The model under review builds one solid part; all positions refer to its coordinate system, in mm. A direction names the side the tool comes from. Round coordinates to 2 decimals unless told otherwise and drop trailing zeros. Loops run counter-clockwise (first coordinate to the right, second up) from the corner with the lowest first, then second, coordinate; pieces in that order, holes last. Notation, with made-up numbers: (22, -29.5) -> (30, -29.5) arc R30 cw to (30, 4.5) -> close; hole circle Ø8 at (81.25, -39). An arc over 180 degrees is marked (long way). Write each question's results on one line, items separated by ' | '. Start each with the question number.
Item 1: Tool access review of faces 4 (the flat face through (0, -10.9, 5)), 5 (the flat face through (0, -15.9, 3)), 6 (the flat face through (11, -12, 0)), 7 (the cylindrical face through (33.831, -23.126, -13.546)): name each direction out of +Z, -Z, +X, -X, +Y, -Y from which nothing blocks a thin tool from reaching the whole face with its end or side.
Item 2: Clearance check with flat-ended pins moving along their axes: pin 1 Ø2 at (x, y) = (26, 6) entering from +Z; pin 2 Ø3.5 at (x, y) = (-24.89, -5) entering from -Z; pin 3 Ø6 at (x, y) = (2.5, -14) entering from +Z; pin 4 Ø8 at (x, y) = (6, 4.5) entering from -Z. State where each tip first meets the part, or that it passes through.
Item 3: We need section D-D (x = 44). Give the boundary of the cut face in (y, z), and give its area (3 significant figures).
Item 4: Mouldability with a two-part tool opening along Z and no side actions: class faces 1 (the flat face through (-24, -7, 4)), 2 (the cylindrical face through (33.831, -23.126, 31.754)), 3 (the flat face through (2, -14.2, -3)) as pulls with the +Z half, pulls with the -Z half, needs draft (parallel to the pull), parting line crosses it, or undercut.
Item 5: We need section C-C (y = 12.5). Give the boundary of the cut face in (x, z), and give its area (3 significant figures).
Item 6: We need section B-B (x = 24.89). Give the boundary of the cut face in (y, z), and give its area (3 significant figures).
Item 7: We need section A-A (x = -9.5). Give the boundary of the cut face in (y, z).
Item 8: For L1, parallel to Y at x = 24.89, z = 5.7; L2, parallel to Y at x = -24.89, z = 3.25; L3, parallel to Z at x = 45, y = 3, list the stretches that pass through material, from the lowest coordinate up. Write a range as from..to.
Autodesk Inventor part; units mm, degrees
ref_plane "YZ Plane" through (0, 0, 0) normal (1, 0, 0) x (0, 1, 0)
ref_plane "XZ Plane" through (0, 0, 0) normal (0, 1, 0) x (-1, 0, 0)
ref_plane "XY Plane" through (0, 0, 0) normal (0, 0, 1) x (1, 0, 0)
sketch "Szkic1" plane through (0, 0, 0) normal (0, 0, 1) x (1, 0, 0)
  line L0 (20.3, -9.9) -> (-20.3, -9.9)
  line L1 (-20.3, -9.9) -> (-20.3, 9.9)
  line L2 (-20.3, 9.9) -> (20.3, 9.9)
  line L3 (20.3, 9.9) -> (20.3, -9.9)
  line L4 (20.3, -9.9) -> (-20.3, 9.9) construction
  line L5 (-20.3, -9.9) -> (20.3, 9.9) construction
  line L6 (21.3, 10.9) -> (-21.3, 10.9)
  line L7 (-21.3, 10.9) -> (-21.3, -10.9)
  line L8 (-21.3, -10.9) -> (21.3, -10.9)
  line L9 (21.3, -10.9) -> (21.3, 10.9)
  line L10 (0, 0) -> (24.89, 0)
  line L11 (24.89, 0) -> (24.89, 5)
  line L12 (24.89, 5) -> (24.89, -5)
  line L13 (0, 0) -> (-24.89, 0)
  line L14 (-24.89, 5) -> (-24.89, 0)
  line L15 (-24.89, 0) -> (-24.89, -5)
  circle A0 centre (-24.89, 5) radius 1.621
  circle A1 centre (-24.89, -5) radius 1.621
  circle A2 centre (24.89, -5) radius 1.621
  circle A3 centre (24.89, 5) radius 1.621
  line L16 (-26.511, 5) -> (-31.511, 5)
  line L17 (26.511, 5) -> (31.511, 5)
  line L18 (0, 10.9) -> (0, 15.9)
  line L19 (0, 15.9) -> (-16.6819, 15.9)
  line L20 (0, -10.9) -> (0, -15.9)
  line L21 (0, -15.9) -> (-16.6819, -15.9)
  line L22 (-31.511, -5.7364) -> (-31.511, 5.7364)
  line L23 (0, 15.9) -> (31.511, 15.9)
  line L24 (31.511, 15.9) -> (31.511, -15.9)
  line L25 (0, -15.9) -> (31.511, -15.9)
  arc A4 (58.9078, 0) -> (31.511, 15.9) centre (29.1703, -19.6864) ccw
  arc A5 (29.1703, -29.1056) -> (15.7555, -15.9) centre (13.2559, -31.8556) ccw
  line L26 (29.1703, -29.1056) -> (58.9078, 0)
  circle A6 centre (-16.6819, 0) radius 15.9
  arc A7 (-32.5353, -15.867) -> (-31.511, -15.9) centre (-31.511, 0) ccw
  point P0 (58.9078, 0)
  dimension "d10" = 3.242
  dimension "d13" = 3.242
  dimension "d0" = 40.6
  dimension "d1" = 19.8
  dimension "d2" = 1
  dimension "d3" = 42.6
  dimension "d4" = 24.89
  dimension "d5" = 5
  dimension "d6" = 10
  dimension "d7" = 24.89
  dimension "d8" = 5
  dimension "d9" = 5
  dimension "d11" = 3.242
  dimension "d12" = 3.242
  dimension "d14" = 5
  dimension "d15" = 5
  dimension "d16" = 5
  dimension "d17" = 5
  dimension "d18" = 6.621
  dimension "d19" = 63.022
  dimension "d20" = 10.9
  dimension "d21" = 0
extrude "Wyciągnięcie proste1" add sketch "Szkic1" along normal blind 10 contours A6 L22 L16 A0 L14 L13 L7 L8 | L8 L20 L21 A6 | L10 L11 A3 L17 L24 L25 L20 L8 L9 | L9 L6 L18 L23 L24 L17 A3 L11 L10 | L13 L14 A0 L16 L22 A6 L6 L7 | A6 L22 | A6 L19 L18 L6 | L25 L24 A4 L26 A5
sketch "Szkic2" plane through (0, 0, 10) normal (0, 0, 1) x (1, 0, 0)
  arc A0 (29.1703, -29.1056) -> (15.7555, -15.9) centre (13.2559, -31.8556) ccw
  line L0 (29.1703, -29.1056) -> (58.9078, 0)
  arc A1 (58.9078, 0) -> (31.511, 15.9) centre (29.1703, -19.6864) ccw
  line L1 (29.1703, -29.1056) -> (58.9078, 0)
  arc A2 (29.1703, -29.1056) -> (15.7555, -15.9) centre (13.2559, -31.8556) ccw
  line L2 (27.3214, -23.9188) -> (55.8385, 3.9923)
  line L3 (31.511, 15.9) -> (-16.6819, 15.9)
  arc A3 (-16.6819, 15.9) -> (-16.6819, -15.9) centre (-16.6819, 0) ccw
  line L4 (-16.6819, -15.9) -> (15.7555, -15.9)
  point P0 (0, 0)
  dimension "d24" = 5
extrude "Wyciągnięcie proste2" add sketch "Szkic2" along normal blind 20 contours A0 L2 A1 L0
sketch "Szkic3" plane through (0, 0, 0) normal (0, 0, -1) x (-1, 0, 0)
  line L0 (-27.3214, -23.9188) -> (-55.8385, 3.9923)
  line L1 (-29.1703, -29.1056) -> (-58.9078, 0)
  arc A0 (-15.7555, -15.9) -> (-29.1703, -29.1056) centre (-13.2559, -31.8556) ccw
  arc A1 (-31.511, 15.9) -> (-58.9078, 0) centre (-29.1703, -19.6864) ccw
  line L2 (-29.1703, -29.1056) -> (-58.9078, 0)
  line L3 (16.6819, -15.9) -> (-15.7555, -15.9)
  arc A2 (16.6819, -15.9) -> (16.6819, 15.9) centre (16.6819, 0) ccw
  line L4 (-31.511, 15.9) -> (16.6819, 15.9)
  point P0 (0, 0)
  point P1 (-55.8385, 3.9923)
extrude "Wyciągnięcie proste3" add sketch "Szkic3" along normal blind 20 contours A0 L1 A1 L0
sketch "Szkic9" plane through (0, 0, 30) normal (0, 0, 1) x (1, 0, 0)
  arc A0 (29.1703, -29.1056) -> (27.3214, -23.9188) centre (13.2559, -31.8556) ccw
  line L0 (29.1703, -29.1056) -> (58.9078, 0)
  arc A1 (58.9078, 0) -> (55.8385, 3.9923) centre (29.1703, -19.6864) ccw
  line L1 (55.8385, 3.9923) -> (27.3214, -23.9188)
  point P0 (0, 0)
extrude "Wyciągnięcie proste5" add sketch "Szkic9" along normal blind 11.3
sketch "Szkic10" plane through (58.9078, 0, -20) normal (0.6995, -0.7147, 0) x (0.7147, 0.6995, 0)
  line L0 (-41.6107, 0) -> (-41.6107, 61.3)
  line L1 (0, 0) -> (-41.6107, 0)
  line L2 (0, 0) -> (0, 61.3)
  line L3 (-41.6107, 61.3) -> (0, 61.3)
  point P0 (-42.099, 20)
  point P1 (-33.6107, 8)
  point P2 (-8, 8)
  point P3 (-33.6107, 53.3)
  point P4 (-8, 53.3)
  dimension "d60" = 8
  dimension "d61" = 8
  dimension "d62" = 8
  dimension "d63" = 8
  dimension "d64" = 8
  dimension "d65" = 8
  dimension "d66" = 8
  dimension "d67" = 8
hole "Otwór2" at (34.8876, -23.5098, -12) at (53.1905, -5.5958, -12) at (34.8876, -23.5098, 33.3) at (53.1905, -5.5958, 33.3) direction (-0.6995, 0.7147, 0) diameter 3.242 end through all
sketch "Szkic12" plane through (55.8385, 3.9923, 0) normal (-0.6995, 0.7147, 0) x (0.7147, 0.6995, 0)
  circle A0 centre (-34.2097, 12) radius 1.621
  circle A1 centre (-8.599, 12) radius 1.621
  line L0 (0, 0) -> (-39.9031, 0)
  line L1 (0, 0) -> (0, 20)
  line L2 (-39.9031, 20) -> (0, 20)
  line L3 (-39.9031, 0) -> (-39.9031, 20)
  circle A2 centre (-34.2097, -33.3) radius 1.621
  circle A3 centre (-8.599, -33.3) radius 1.621
  line L4 (-39.9031, -10) -> (0, -10)
  line L5 (-39.9031, -10) -> (-39.9031, -41.3)
  line L6 (0, -41.3) -> (-39.9031, -41.3)
  line L7 (0, -10) -> (0, -41.3)
  circle A4 centre (-8.599, 12) radius 1.621
  circle A5 centre (-8.599, 12) radius 3.5
  circle A6 centre (-34.2097, 12) radius 3.5
  circle A7 centre (-34.2097, -33.3) radius 3.5
  circle A8 centre (-8.599, -33.3) radius 3.5
  point P0 (-42.698, 0)
  dimension "d77" = 7
  dimension "d78" = 7
  dimension "d79" = 7
  dimension "d80" = 7
extrude "Wyciągnięcie proste6" cut sketch "Szkic12" against normal blind 3 contours A0 | A1 | A2 | A3 | A5 | A6 | A7 | A8
sketch "Szkic15" plane through (0, 0, 0) normal (0, 0, -1) x (-1, 0, 0)
  line L0 (-55.8385, 3.9923) -> (-27.3214, -23.9188)
  arc A0 (-15.7555, -15.9) -> (-27.3214, -23.9188) centre (-13.2559, -31.8556) ccw
  line L1 (16.6819, -15.9) -> (-15.7555, -15.9)
  arc A1 (16.6819, -15.9) -> (16.6819, 15.9) centre (16.6819, 0) ccw
  line L2 (-31.511, 15.9) -> (16.6819, 15.9)
  arc A2 (-31.511, 15.9) -> (-55.8385, 3.9923) centre (-29.1703, -19.6864) ccw
  circle A3 centre (24.89, 5) radius 1.621
  circle A4 centre (24.89, -5) radius 1.621
  line L3 (-21.3, 10.9) -> (-21.3, -10.9)
  line L4 (21.3, 10.9) -> (-21.3, 10.9)
  line L5 (21.3, -10.9) -> (21.3, 10.9)
  line L6 (-21.3, -10.9) -> (21.3, -10.9)
  circle A5 centre (-24.89, -5) radius 1.621
  circle A6 centre (-24.89, 5) radius 1.621
  arc A7 (16.6819, -13.9) -> (16.6819, 13.9) centre (16.6819, 0) ccw
  line L7 (16.6819, -13.9) -> (-15.9066, -13.9)
  arc A8 (-15.9066, -13.9) -> (-27.6497, -20.799) centre (-13.2559, -31.8556) ccw
  line L8 (-27.6497, -20.799) -> (-53.0395, 4.0513)
  arc A9 (-31.4443, 13.9) -> (-53.0395, 4.0513) centre (-29.1703, -19.6864) ccw
  line L9 (-31.4443, 13.9) -> (16.6819, 13.9)
  line L10 (-53.0395, 4.0513) -> (-54.4074, 2.5916)
  line L11 (-55.8385, 3.9923) -> (-27.3214, -23.9188)
  line L12 (-27.6497, -20.799) -> (-29.0176, -22.2587)
  point P0 (0, 0)
  dimension "d86" = 2
extrude "Wyciągnięcie proste8" add sketch "Szkic15" along normal blind 3 contours A2 L2 A1 L1 A0 L0 L12 A8 L7 A7 L9 A9 L10
sketch "Szkic17" plane through (0, 0, 10) normal (0, 0, 1) x (1, 0, 0)
  line L0 (27.3214, -23.9188) -> (55.8385, 3.9923)
  arc A0 (55.8385, 3.9923) -> (31.511, 15.9) centre (29.1703, -19.6864) ccw
  line L1 (31.511, 15.9) -> (-16.6819, 15.9)
  arc A1 (-16.6819, 15.9) -> (-16.6819, -15.9) centre (-16.6819, 0) ccw
  line L2 (-16.6819, -15.9) -> (15.7555, -15.9)
  arc A2 (27.3214, -23.9188) -> (15.7555, -15.9) centre (13.2559, -31.8556) ccw
  circle A3 centre (-24.89, 5) radius 1.621
  circle A4 centre (-24.89, -5) radius 1.621
  line L3 (21.3, 10.9) -> (21.3, -10.9)
  line L4 (21.3, -10.9) -> (-21.3, -10.9)
  line L5 (-21.3, -10.9) -> (-21.3, 10.9)
  line L6 (-21.3, 10.9) -> (21.3, 10.9)
  circle A5 centre (24.89, -5) radius 1.621
  circle A6 centre (24.89, 5) radius 1.621
  circle A7 centre (-24.89, -5) radius 3.5
  circle A8 centre (-24.89, 5) radius 1.621
  circle A9 centre (-24.89, 5) radius 3.5
  circle A10 centre (24.89, -5) radius 3.5
  circle A11 centre (24.89, 5) radius 3.5
  point P0 (0, 0)
  dimension "d89" = 7
  dimension "d90" = 7
  dimension "d91" = 7
  dimension "d92" = 7
extrude "Wyciągnięcie proste9" cut sketch "Szkic17" against normal blind 6 contours A7 | A9 | A10 | A11
equation "\"d13\" = d10"
equation "\"d11\" = d10"
equation "\"d12\" = d10"
properties part number "Ramie1_Drukowanie 3D"
Here are the results:
1) face 4: +Z, -Z | face 5: +Z, -Z, -X, -Y | face 6: -Z | face 7: none
2) pin 1: stops at z = 4 | pin 2: stops at z = 0 | pin 3: stops at z = 10 | pin 4: passes through
3) outline: (-14.59, -20) -> (-7.59, -20) -> (-7.59, 0) -> (10.53, 0) -> (10.53, -3) -> (12.75, -3) -> (12.75, 10) -> (-7.59, 10) -> (-7.59, 41.3) -> (-14.59, 41.3) -> close | area: 639 mm2
4) face 1: pulls with the +Z half | face 2: undercut | face 3: pulls with the -Z half
5) outline: (-26.51, -3) -> (-22.76, -3) -> (-22.76, 0) -> (39.03, 0) -> (39.03, -3) -> (44.53, -3) -> (44.53, 10) -> (-26.51, 10) -> close | area: 738 mm2
6) outline: (-20.65, -3) -> (-17.92, -3) -> (-17.92, 0) -> (-6.62, 0) -> (-6.62, 4) -> (-8.5, 4) -> (-8.5, 10) -> (-20.65, 10) -> close; (-3.38, 0) -> (3.38, 0) -> (3.38, 4) -> (1.5, 4) -> (1.5, 10) -> (-1.5, 10) -> (-1.5, 4) -> (-3.38, 4) -> close; (6.62, 0) -> (13.9, 0) -> (13.9, -3) -> (15.9, -3) -> (15.9, 10) -> (8.5, 10) -> (8.5, 4) -> (6.62, 4) -> close | area: 270 mm2
7) outline: (-15.9, -3) -> (-13.9, -3) -> (-13.9, 0) -> (-10.9, 0) -> (-10.9, 10) -> (-15.9, 10) -> close; (10.9, 0) -> (13.9, 0) -> (13.9, -3) -> (15.9, -3) -> (15.9, 10) -> (10.9, 10) -> close
8) L1: y = -20.65..-8.5, -1.5..1.5, 8.5..15.9 | L2: y = -13.62..-6.62, -3.38..3.38, 6.62..13.62 | L3: z = 0..10
